Read the model definition and answer for the solid it produces. Units are mm, in the model's axes. Face numbers are marked on the shaded views. A direction names the side the tool comes from. Coordinates: 2 decimals unless noted, no trailing zeros. Loops run counter-clockwise (first coordinate to the right, second up) from the corner with the lowest first, then second, coordinate; pieces in that order, holes last.
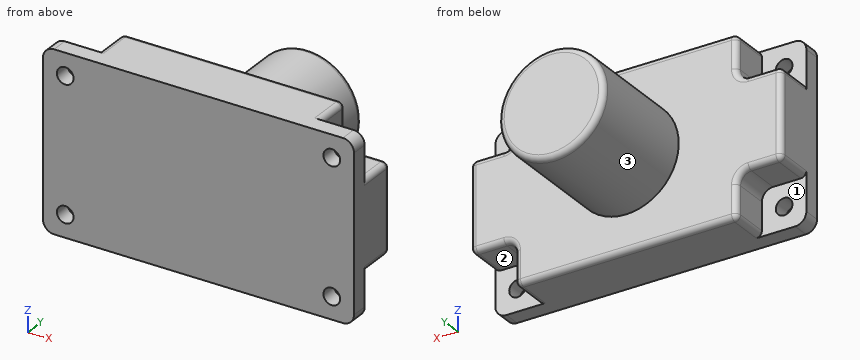
from build123d import *

# Parameters (mm, degrees)
CROQUIS1_W              = 56
CROQUIS1_H              = 32
SALIENTE_EXTRUIR1_DEPTH = 10
CROQUIS2_R              = 9.5
SALIENTE_EXTRUIR2_DEPTH = 21
CROQUIS3_W              = 8
CROQUIS3_H              = 8
CORTAR_EXTRUIR1_DEPTH   = 7
CROQUIS4_R              = 1.5
CORTAR_EXTRUIR2_DEPTH   = 71.313583325
REDONDEO1_R             = 2
REDONDEO2_R             = 1
REDONDEO3_R             = 1
REDONDEO4_R             = 1


with BuildPart() as part:
    # Croquis1 → Saliente-Extruir1 (new body)
    with BuildSketch(Plane(origin=(0, 0, 0), x_dir=(1, 0, 0), z_dir=(0, 1, 0))):
        with Locations((28, -16)):
            Rectangle(CROQUIS1_W, CROQUIS1_H)
    extrude(amount=SALIENTE_EXTRUIR1_DEPTH)

    # Croquis2 → Saliente-Extruir2 (add)
    with BuildSketch(Plane(origin=(0, 10, 0), x_dir=(1, 0, 0), z_dir=(0, 1, 0))):
        with Locations(Location((28, -16, 0), (0, 0, 90))):
            Circle(CROQUIS2_R)
    extrude(amount=SALIENTE_EXTRUIR2_DEPTH)

    # Croquis3 → Cortar-Extruir1 (cut)
    with BuildSketch(Plane(origin=(0, 10, 0), x_dir=(1, 0, 0), z_dir=(0, 1, 0))):
        with Locations((52, -28)):
            Rectangle(CROQUIS3_W, CROQUIS3_H)
        with Locations((52, -4)):
            Rectangle(CROQUIS3_W, CROQUIS3_H)
        with Locations((4, -4)):
            Rectangle(CROQUIS3_W, CROQUIS3_H)
        with Locations((4, -28)):
            Rectangle(CROQUIS3_W, CROQUIS3_H)
    extrude(amount=-CORTAR_EXTRUIR1_DEPTH, mode=Mode.SUBTRACT)

    # Croquis4 → Cortar-Extruir2 (cut, through all)
    with BuildSketch(Plane(origin=(0, 3, 0), x_dir=(1, 0, 0), z_dir=(0, 1, 0))):
        with Locations(Location((4, -4, 0), (0, 0, 270))):
            Circle(CROQUIS4_R)
        with Locations(Location((4, -28, 0), (0, 0, 270))):
            Circle(CROQUIS4_R)
        with Locations(Location((52, -28, 0), (0, 0, 270))):
            Circle(CROQUIS4_R)
        with Locations(Location((52, -4, 0), (0, 0, 270))):
            Circle(CROQUIS4_R)
    extrude(amount=-CORTAR_EXTRUIR2_DEPTH, mode=Mode.SUBTRACT)

    # Redondeo1
    redondeo1_edges = [part.edges().sort_by_distance(p)[0] for p in [
        (0, 1.5, 0),
        (56, 1.5, 0),
        (56, 1.5, 32),
        (0, 1.5, 32),
        (8, 6.5, 24),
        (8, 6.5, 8),
        (48, 6.5, 8),
        (48, 6.5, 24),
    ]]
    fillet(redondeo1_edges, radius=REDONDEO1_R)

    # Redondeo2
    redondeo2_edges = [part.edges().sort_by_distance(p)[0] for p in [
        (0, 10, 16),
        (28, 10, 32),
        (56, 10, 16),
        (28, 10, 0),
    ]]
    fillet(redondeo2_edges, radius=REDONDEO2_R)

    # Redondeo3
    redondeo3_edges = [part.edges().sort_by_distance(p)[0] for p in [
        (48, 10, 28.5),
        (8, 10, 3.5),
        (3.5, 10, 24),
        (48.585786438, 10, 7.414213562),
        (48.585786438, 10, 24.585786438),
        (7.414213562, 10, 7.414213562),
        (7.414213562, 10, 24.585786438),
        (8, 10, 28.5),
        (52.5, 10, 24),
        (48, 10, 3.5),
        (3.5, 10, 8),
        (0.292893219, 9.707106781, 24),
        (0.292893219, 9.707106781, 8),
        (8, 9.707106781, 0.292893219),
        (48, 9.707106781, 0.292893219),
        (55.707106781, 9.707106781, 8),
        (55.707106781, 9.707106781, 24),
        (48, 9.707106781, 31.707106781),
        (8, 9.707106781, 31.707106781),
        (8, 6, 32),
        (0, 6, 24),
        (0, 6, 8),
        (8, 6, 0),
        (48, 6, 0),
        (56, 6, 8),
        (48, 6, 32),
        (56, 6, 24),
        (52.5, 10, 8),
    ]]
    fillet(redondeo3_edges, radius=REDONDEO3_R)

    # Redondeo4
    redondeo4_edges = [part.edges().sort_by_distance(p)[0] for p in [
        (28, 31, 25.5),
    ]]
    fillet(redondeo4_edges, radius=REDONDEO4_R)


solid = part.part
Q1. Straight lines are drawn through the part: probe 1 along Y at (x, z) = (30, 2.5); probe 2 along Y at (x, z) = (51.5, 26); probe 3 along Z at (x, y) = (32, 21.5). For each, find the intervals that lie inside material, in ascending order.
Findings below:
probe 1: y = 0 to 10
probe 2: y = 0 to 3
probe 3: z = 7.38 to 24.62
Q2. A cutting plane is placed at B-B (z = 4). Give the vertices of the cut face in (x, y), then the cut area to 3 significant figures.
Findings below:
outline: (0, 0) - (2.5, 0) - (2.5, 3) - (0, 3) - close; (5.5, 0) - (50.5, 0) - (50.5, 3) - (48, 3) - (48, 9) arc R1 ccw to (47, 10) - (9, 10) arc R1 ccw to (8, 9) - (8, 3) - (5.5, 3) - close; (53.5, 0) - (56, 0) - (56, 3) - (53.5, 3) - close
area: 430 mm2
Q3. A cutting plane is placed at C-C (x = 28). Give the vertices of the cut face in (y, z), then the cut area to 3 significant figures.
Findings below:
outline: (0, 0) - (9, 0) arc R1 ccw to (10, 1) - (10, 6.5) - (30, 6.5) arc R1 ccw to (31, 7.5) - (31, 24.5) arc R1 ccw to (30, 25.5) - (10, 25.5) - (10, 31) arc R1 ccw to (9, 32) - (0, 32) - close
area: 718 mm2
Q4. A cutting plane is placed at A-A (x = 52). Give the vertices of the cut face in (y, z), then the cut area to 3 significant figures.
Findings below:
outline: (0, 0) - (3, 0) - (3, 2.5) - (0, 2.5) - close; (0, 5.5) - (3, 5.5) - (3, 8) - (9, 8) arc R1 ccw to (10, 9) - (10, 23) arc R1 ccw to (9, 24) - (3, 24) - (3, 26.5) - (0, 26.5) - close; (0, 29.5) - (3, 29.5) - (3, 32) - (0, 32) - close
area: 190 mm2
Q5. A cutting plane is placed at D-D (z = 16). Give the vertices of the cut face in (x, y), then the cut area to 3 significant figures.
Findings below:
outline: (0, 0) - (56, 0) - (56, 9) arc R1 ccw to (55, 10) - (37.5, 10) - (37.5, 30) arc R1 ccw to (36.5, 31) - (19.5, 31) arc R1 ccw to (18.5, 30) - (18.5, 10) - (1, 10) arc R1 ccw to (0, 9) - close
area: 958 mm2
Q6. Flat-ended cylindrical pins translate along their axes: pin 1 Ø10 at (x, z) = (42, 21) entering from +Y; pin 2 Ø4 at (x, y) = (52, 7) entering from -Z; pin 3 Ø2.5 at (x, y) = (53.5, 4.5) entering from +Z. Find the tip coordinate at first contact, or state that the pin passes through.
Findings below:
pin 1: stops at y = 10
pin 2: stops at z = 8
pin 3: stops at z = 24
Q7. Which of the six approach directions +Z, -Z, +X, -X, +Y, -Y give full straight-line access (tool end or side, diameter ignored) to the marked faces 1, 2 and 3?
Findings below:
face 1: -Z, -X, +Y
face 2: -Z, +X, +Y
face 3: +Y
